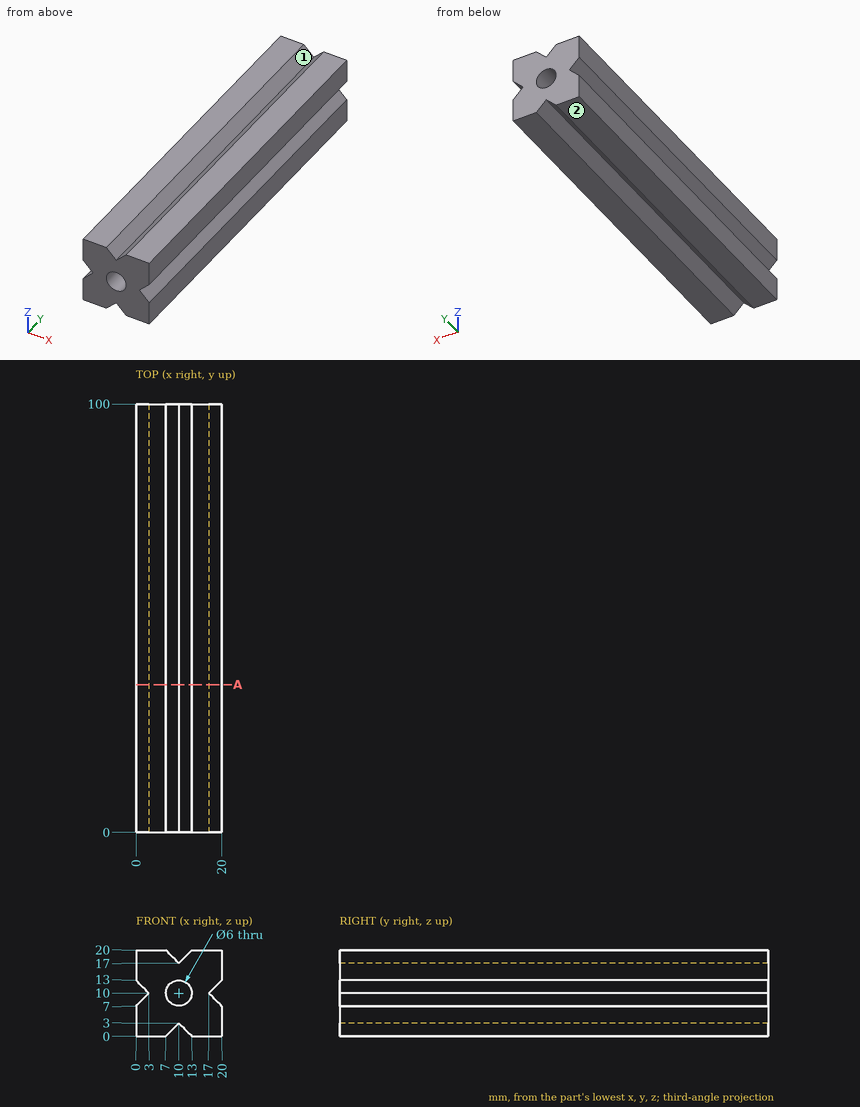
Part print with two shaded views. Sizes in mm from the minimum x, y, z corner. Round coordinates to 2 decimals unless told otherwise and drop trailing zeros. Loops run counter-clockwise (first coordinate to the right, second up) from the corner with the lowest first, then second, coordinate; pieces in that order, holes last. Notation, with made-up numbers: M -30.5,42 L -14.5,42 A16 cw -14.5,69 Z; hole C -33,-18.75 d1. An arc over 180 degrees is marked long. Return JSON: item names as keys, results as strings. Group by question number.
(1) Mould opens along X. For the marked faces 1 and 2 say: +X half, -X half, draft (parallel to the pull), parting line (faces both ways), or undercut.
(2) Saw through at A-A, the plane y = 34.5. List the corners of the cut face in (x, z), and give its area (3 significant figures).
(3) Wall check: probe 1 along X at (y, z) = (41, 10); probe 2 along Z at (x, y) = (8.75, 77.5); probe 3 along Z at (x, y) = (9.25, 94.5). Give the ranges that are in metal, low to high. Write a range as [from, to].
(4) Drop flat-ended pins along their axis: P1, Ø2, axis at y = 34, z = 11.5, coming from the +X side; P2, Ø1, axis at x = 10.5, y = 37, coming from the -Z side. Give the stop position or say it passes through.
Answer list:
{
 "1": {"face 1": "undercut", "face 2": "draft"},
 "2": {"outline": "M 0,0 L 7,0 L 10,3 L 13,0 L 20,0 L 20,7 L 17,10 L 20,13 L 20,20 L 13,20 L 10,17 L 7,20 L 0,20 L 0,13 L 3,10 L 0,7 Z; hole C 10,10 d6", "area": "336 mm2"},
 "3": {"probe 1": "[3, 7], [13, 17]", "probe 2": "[1.75, 7.27], [12.73, 18.25]", "probe 3": "[2.25, 7.1], [12.9, 17.75]"},
 "4": {"P1": "x = 19.5", "P2": "z = 2"}
}
